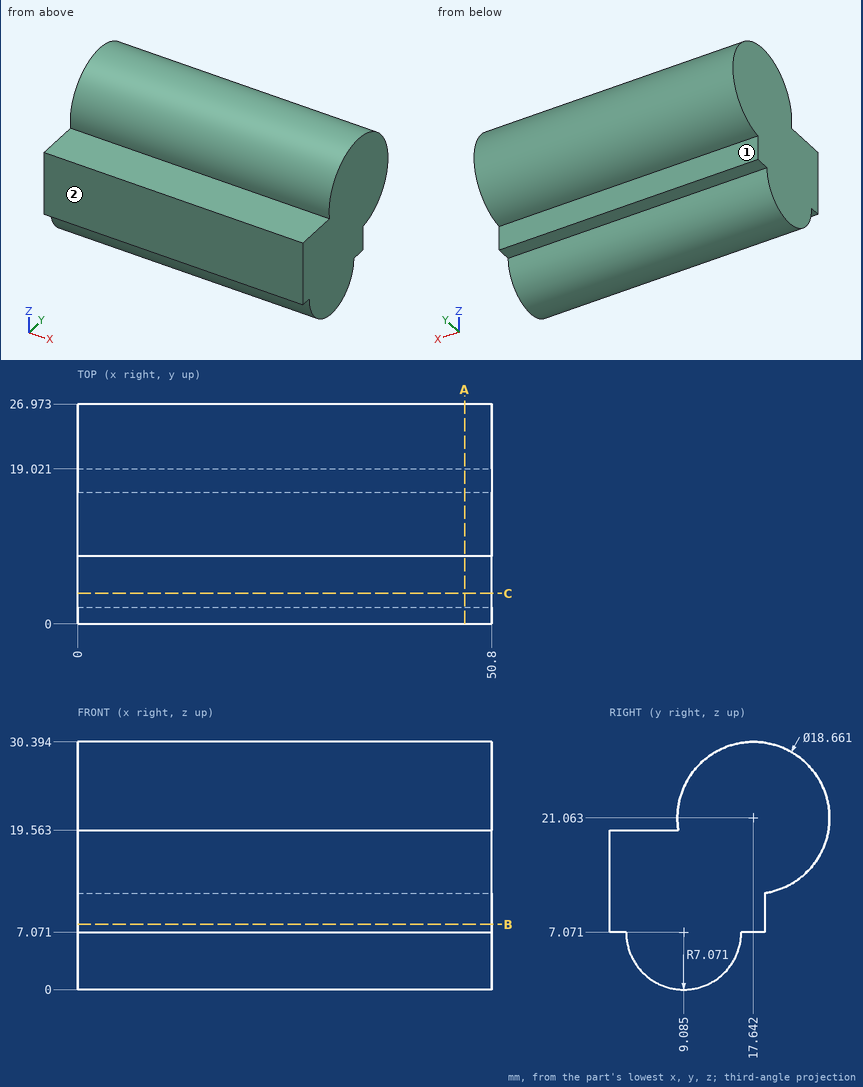
Verification items for this drawing (mm, ordinates from the low corner). A direction names the side the tool comes from. Coordinates: 2 decimals unless noted, no trailing zeros. Write each loop counter-clockwise with the first axis right and the second up, starting at its lowest first coordinate (ties: lowest second). Pieces come first, ordered by that corner, then holes. Notation, with made-up numbers: M 39.5,63.5 L 87.5,63.5 A18 cw 87.5,90.5 Z; hole C 7,34.25 d2. An arc over 180 degrees is marked long. Answer as CSV lines item,"result".
Q1. Cross-section at C-C (y = 3.75). Record the boundary of the cut face in (x, z).
Check result:
outline,"M 0,2.43 L 50.8,2.43 L 50.8,19.56 L 0,19.56 Z"
Q2. Go/stop test with flat-tipped pins: pin 1 (3 mm diameter, centred on x = 18, z = 8, fed in from +Y); pin 2 (1 mm diameter, centred on x = 34, y = 8, fed in from -Z); pin 3 (10 mm diameter, centred on x = 6, y = 8.5, fed in from +Z). Record where each tip stops, or that it passes through.
Check result:
pin 1,"y = 19.02"
pin 2,"z = 0.02"
pin 3,"z = 29.42"
Q3. Set-up check for the marked faces 1 and 2: record each of +Z, -Z, +X, -X, +Y, -Y from which the full face is reachable in a straight line by a thin tool's end or side.
Check result:
face 1,"-Z, +X, -X, +Y"
face 2,"+Z, -Z, +X, -X, -Y"
Q4. Cross-section at B-B (z = 8). Record the boundary of the cut face in (x, y), then the cut area to 3 significant figures.
Check result:
outline,"M 0,0 L 50.8,0 L 50.8,19.02 L 0,19.02 Z"
area,"966 mm^2"
Q5. Material ranges on probe 1 along Y at (x, z) = (46.5, 9); probe 2 along Z at (x, y) = (26.5, 1.5); probe 3 along Y at (x, z) = (3, 18.5) (1 decimal), recorded low to high. Write a range as from..to.
Check result:
probe 1,"0..19.02"
probe 2,"7.07..19.56"
probe 3,"0..26.6"
Q6. Cross-section at A-A (x = 47.5). Record the boundary of the cut face in (y, z) (1 decimal).
Check result:
outline,"M 0,7.1 L 2,7.1 A7.1 ccw 16.2,7.1 L 19,7.1 L 19,11.8 A9.3 ccw long 8.4,19.6 L 0,19.6 Z"
